from build123d import *

# Parameters (mm, degrees)
SKETCH1_R                                 = 2.38125
EXTRUDE1_DEPTH                            = 15.875
F_4_40_TAPPED_HOLE1_D                     = 2.2606
F_4_40_TAPPED_HOLE1_DEPTH                 = 7.62
F_4_40_TAPPED_HOLE1_CBORE_D               = 2.8448
F_4_40_TAPPED_HOLE1_CBORE_DEPTH           = 5.588
F_4_40_TAPPED_HOLE1_TIP                   = 0.679152758
F_4_40_TAPPED_HOLE1_ON_FACE_2_D           = 2.2606
F_4_40_TAPPED_HOLE1_ON_FACE_2_DEPTH       = 7.62
F_4_40_TAPPED_HOLE1_ON_FACE_2_CBORE_D     = 2.8448
F_4_40_TAPPED_HOLE1_ON_FACE_2_CBORE_DEPTH = 5.588
F_4_40_TAPPED_HOLE1_ON_FACE_2_TIP         = 0.679152758
CHAMFER1_SIZE                             = 0.127
CHAMFER1_SIZE2                            = 0.720252791


with BuildPart() as part:
    # Sketch1 → Extrude1 (new body)
    with BuildSketch(Plane(origin=(0, 0, 0), x_dir=(1, 0, 0), z_dir=(0, 1, 0))):
        with Locations(Location((0, 0, 0), (0, 0, 270))):  # turned: the seam where the file's is
            Circle(SKETCH1_R)
    extrude(amount=EXTRUDE1_DEPTH)

    # #4-40 Tapped Hole1
    with Locations(Plane.ZX.offset(15.875)):
        with Locations((0, 0)):
            CounterBoreHole(F_4_40_TAPPED_HOLE1_D / 2, F_4_40_TAPPED_HOLE1_CBORE_D / 2, F_4_40_TAPPED_HOLE1_CBORE_DEPTH, depth=F_4_40_TAPPED_HOLE1_DEPTH)
            with Locations((0, 0, -(F_4_40_TAPPED_HOLE1_DEPTH + F_4_40_TAPPED_HOLE1_TIP / 2))):  # 118° drill point
                Cone(0, F_4_40_TAPPED_HOLE1_D / 2, F_4_40_TAPPED_HOLE1_TIP, mode=Mode.SUBTRACT)

    # #4-40 Tapped Hole1 on face 2
    with Locations(Plane(origin=(0, 0, 0), x_dir=(0, 0, -1), z_dir=(0, -1, 0))):
        with Locations((0, 0)):
            CounterBoreHole(F_4_40_TAPPED_HOLE1_ON_FACE_2_D / 2, F_4_40_TAPPED_HOLE1_ON_FACE_2_CBORE_D / 2, F_4_40_TAPPED_HOLE1_ON_FACE_2_CBORE_DEPTH, depth=F_4_40_TAPPED_HOLE1_ON_FACE_2_DEPTH)
            with Locations((0, 0, -(F_4_40_TAPPED_HOLE1_ON_FACE_2_DEPTH + F_4_40_TAPPED_HOLE1_ON_FACE_2_TIP / 2))):  # 118° drill point
                Cone(0, F_4_40_TAPPED_HOLE1_ON_FACE_2_D / 2, F_4_40_TAPPED_HOLE1_ON_FACE_2_TIP, mode=Mode.SUBTRACT)

    # Chamfer1
    chamfer1_edges = [part.edges().sort_by_distance(p)[0] for p in [
        (0, 15.875, -1.4224),
    ]]
    chamfer1_side = [part.faces().sort_by_distance(p)[0] for p in [
        (0, 13.081, -1.4224),
    ]]
    chamfer(chamfer1_edges, length=CHAMFER1_SIZE, length2=CHAMFER1_SIZE2, reference=chamfer1_side[0])


solid = part.part
Here's how the part is built. I have some questions about the finished solid (model axes, mm). A direction names the side the tool comes from. Give positions to 0.01 mm unless a question says otherwise; leave off trailing zeros. Write each loop counter-clockwise with the first axis right and the second up, starting at its lowest first coordinate (ties: lowest second). Pieces come first, ordered by that corner, then holes. Notation, with made-up numbers: (52.25, 30) -> (102.25, 30) arc R12 cw to (102.25, 36) -> close; hole circle Ø11 at (-18.75, -33). An arc over 180 degrees is marked (long way). Use one line per item in the form item = value. Start each with the question number.
1. Thinking about a two-plate mould opening in X: for faces 3 (the face through (-1.45, 7.83, -1.89)), 4 (the face through (-1.39, 2.75, 0.31)), 5 (the face through (-2, 0, 0)), which applies, +X half, -X half, draft (parallel to the pull), parting line (faces both ways), or undercut?
2. Imagine slicing it at C-C on y = 9. List the corners of the cut face in (x, z) for me.
3. If I drill on L1, parallel to X at y = 13, z = 0; L2, parallel to X at y = 8.9, z = 0; L3, parallel to Z at x = 0.95, y = 14, over which ranges is the centre line in solid material (lowest first)?
4. Imagine slicing it at D-D on y = 13.75. List the corners of the cut face in (x, z) for me, plus the area to 3 significant figures.
5. On a 3-axis mill with a long thin cutter (end or side, diameter ignored), from which of +Z, -Z, +X, -X, +Y, -Y can I reach the whole of each face in a straight line? I mean faces 1 (the face through (-1.39, 13.06, -0.31)), 2 (the face through (-1.103, 6.618, -0.245)). Say none if no direction works.
6. Will these pins go through, and if not, where does the flat tip stop? pin 1 Ø2.5 at (x, z) = (0.5, 0) entering from +Y; pin 2 Ø1.8 at (x, z) = (0, 0) entering from -Y; pin 3 Ø2.5 at (x, z) = (0, 0) entering from +Y.
Entries:
q1.face_3 = parting line
q1.face_4 = undercut
q1.face_5 = draft
q2.outline = circle Ø4.76 at (0, 0); hole circle Ø2.26 at (0, 0)
q3.L1 = -2.38 to -1.42, 1.42 to 2.38
q3.L2 = -2.38 to -1.13, 1.13 to 2.38
q3.L3 = -2.18 to -1.06, 1.06 to 2.18
q4.outline = circle Ø4.76 at (0, 0); hole circle Ø2.84 at (0, 0)
q4.area = 11.5 mm²
q5.face_1 = +Y
q5.face_2 = -Y
q6.pin_1 = 15.81
q6.pin_2 = 7.76
q6.pin_3 = 10.29
